Autodesk Inventor part; units mm, degrees
ref_plane "YZ Plane" through (0, 0, 0) normal (1, 0, 0) x (0, 1, 0)
ref_plane "XZ Plane" through (0, 0, 0) normal (0, 1, 0) x (-1, 0, 0)
ref_plane "XY Plane" through (0, 0, 0) normal (0, 0, 1) x (1, 0, 0)
sketch "Sketch1" plane through (0, 0, 0) normal (0, 1, 0) x (-1, 0, 0)
  line L0 (-13, 11) -> (13, 11)
  line L1 (13, 11) -> (13, -11)
  line L2 (13, -11) -> (-13, -11)
  line L3 (-13, -11) -> (-13, 11)
  line L4 (-13, 11) -> (13, -11) construction
  line L5 (-4.3445, -6.7829) -> (-10.3445, -6.7829) construction
  line L6 (-4.3445, -4.7829) -> (-10.3445, -4.7829)
  line L7 (-10.3445, -8.7829) -> (-4.3445, -8.7829)
  arc A0 (-4.3445, -8.7829) -> (-4.3445, -4.7829) centre (-4.3445, -6.7829) ccw
  arc A1 (-10.3445, -4.7829) -> (-10.3445, -8.7829) centre (-10.3445, -6.7829) ccw
  line L8 (0, 0) -> (1.6306, 0)
  line L9 (0, 0) -> (1.2871, 0)
  line L10 (10.1555, 6.7829) -> (4.1555, 6.7829) construction
  line L11 (10.1555, 4.7829) -> (4.1555, 4.7829)
  line L12 (4.1555, 8.7829) -> (10.1555, 8.7829)
  arc A2 (10.1555, 4.7829) -> (10.1555, 8.7829) centre (10.1555, 6.7829) ccw
  arc A3 (4.1555, 8.7829) -> (4.1555, 4.7829) centre (4.1555, 6.7829) ccw
  point P0 (-7.3445, -6.7829)
  point P1 (7.1555, 6.7829)
  dimension "d0" = 26
  dimension "d1" = 22
  dimension "d5" = 6
  dimension "d6" = 4
  dimension "d19" = 6
  dimension "d20" = 4
  dimension "d21" = 14.5
extrude "Extrusion1" add sketch "Sketch1" along normal blind 2.2
ref_plane "Work Plane1" through (-13, 0, 0) normal (0, 0, 1) x (1, 0, 0)
properties part number "riser1.7mm"
Geometry check sheet. Reference: the model listing, model coordinates, mm. A direction names the side the tool comes from. Give positions to 0.01 mm unless a question says otherwise; leave off trailing zeros. Order: outer loops, then holes, each group sorted by start corner. A loop starts at its lowest first (then second) coordinate and runs counter-clockwise, first axis right, second up. Notation, with made-up numbers: (-0.75, -36.75) - (31.25, -36.75) arc R12 cw to (31.25, -26.75) - close; hole circle Ø4 at (-40, 47.25). An arc over 180 degrees is marked (long way). Write item = value, one per line. Start each with the question number.
1) Access from +Z, -Z, +X, -X, +Y, -Y to the whole of each face (thin tool, end or side, straight path). Record for faces 1 (the cylindrical face through (12.344, 1.085, -6.827)), 2 (the flat face through (13, 1, 0)).
2) Section check C-C (y = 1.65). Enter the section's corners in (x, z), then the cut area to 3 significant figures.
3) Section check A-A (x = 6.5). Enter the section's corners in (y, z), then the cut area to 3 significant figures.
4) Scan lines: L1, parallel to Z at x = 6.5, y = 1.65; L2, parallel to Z at x = -5.5, y = 1.45; L3, parallel to X at y = 1.35, z = -8. Record each from-to range of solid material in increasing order.
5) Draft check along X on faces 3 (the flat face through (0, 1, -11)), 4 (the flat face through (-7, 1, 8.783)), 5 (the cylindrical face through (-2.156, 1.085, 6.739)), 6 (the flat face through (-13, 1, 0)). Enter one of: released by +X, released by -X, zero draft, split by the parting line, or undercut.
6) Section check B-B (z = 6.75). Enter the section's corners in (x, y), then the cut area to 3 significant figures.
Geometry check:
q1.face_1 = +Y, -Y
q1.face_2 = +Z, -Z, +X, +Y, -Y
q2.outline = (-13, -11) - (13, -11) - (13, 11) - (-13, 11) - close; hole (-10.16, 4.78) - (-4.16, 4.78) arc R2 ccw to (-4.16, 8.78) - (-10.16, 8.78) arc R2 ccw to start; hole (4.34, -8.78) - (10.34, -8.78) arc R2 ccw to (10.34, -4.78) - (4.34, -4.78) arc R2 ccw to start
q2.area = 499 mm2
q3.outline = (0, -11) - (2.2, -11) - (2.2, -8.78) - (0, -8.78) - close; (0, -4.78) - (2.2, -4.78) - (2.2, 11) - (0, 11) - close
q3.area = 39.6 mm2
q4.L1 = -11 to -8.78, -4.78 to 11
q4.L2 = -11 to 4.78, 8.78 to 11
q4.L3 = -13 to 2.76, 11.93 to 13
q5.face_3 = zero draft
q5.face_4 = undercut
q5.face_5 = undercut
q5.face_6 = released by -X
q6.outline = (-13, 0) - (-12.16, 0) - (-12.16, 2.2) - (-13, 2.2) - close; (-2.16, 0) - (13, 0) - (13, 2.2) - (-2.16, 2.2) - close
q6.area = 35.2 mm2
